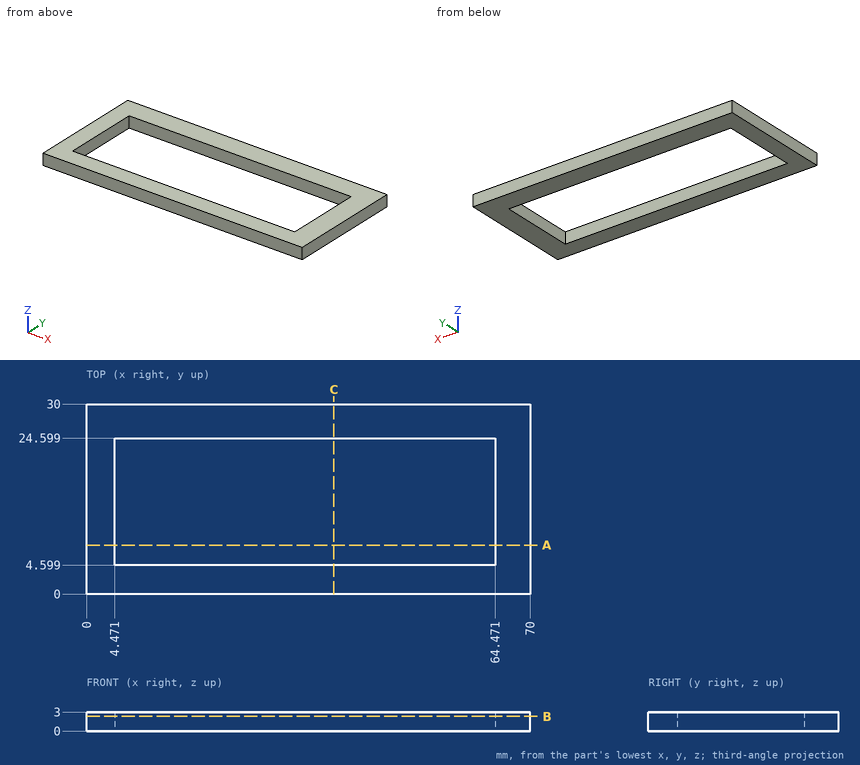
Part print with two shaded views. Sizes in mm from the minimum x, y, z corner. Give positions to 0.01 mm unless a question says otherwise; leave off trailing zeros. Loops run counter-clockwise (first coordinate to the right, second up) from the corner with the lowest first, then second, coordinate; pieces in that order, holes last. Notation, with made-up numbers: (43, 31) -> (68, 31) arc R19 ccw to (68, 55) -> close; hole circle Ø5 at (89.25, -32). An arc over 180 degrees is marked (long way). One line per question, with ' | ' between items.
Q1. Cut at C-C, the plane x = 39. Write the cut outline in (y, z).
Filled sheet:
outline: (0, 0) -> (4.6, 0) -> (4.6, 3) -> (0, 3) -> close; (24.6, 0) -> (30, 0) -> (30, 3) -> (24.6, 3) -> close
Q2. Cut at B-B, the plane z = 2.35. Write the cut outline in (x, y).
Filled sheet:
outline: (0, 0) -> (70, 0) -> (70, 30) -> (0, 30) -> close; hole (4.47, 4.6) -> (64.47, 4.6) -> (64.47, 24.6) -> (4.47, 24.6) -> close
Q3. Cut at A-A, the plane y = 7.75. Write the cut outline in (x, z), plus the area to 3 significant figures.
Filled sheet:
outline: (0, 0) -> (4.47, 0) -> (4.47, 3) -> (0, 3) -> close; (64.47, 0) -> (70, 0) -> (70, 3) -> (64.47, 3) -> close | area: 30.0 mm²
Q4. Drop a flat-ended pin along its axis: pin 1 (6 mm diameter, centred on x = 34, y = 21, fed in from -Z). Give the stop position or say it passes through.
Filled sheet:
pin 1: passes through
Q5. Drill centre lines: line 1 along X through (y, z) = (7, 1.25); line 2 along Y through (x, z) = (13, 1.75). Where is each one in solid material? Low to high. Write a range as [from, to].
Filled sheet:
line 1: x = [0, 4.47], [64.47, 70] | line 2: y = [0, 4.6], [24.6, 30]
